The listing builds one solid part. Answer for the finished solid, in the listing's coordinates (mm). Face numbers are marked on the shaded views. A direction names the side the tool comes from. Give positions to 0.01 mm unless a question says otherwise; leave off trailing zeros. Loops run counter-clockwise (first coordinate to the right, second up) from the corner with the lowest first, then second, coordinate; pieces in that order, holes last. Notation, with made-up numbers: M 79.25,87 L 131.25,87 A16 cw 131.25,100 Z; hole C 78,57.25 d3. An arc over 180 degrees is marked long. One line per item, written item: value. Start each with the question number.
Q1. The mould has two halves that part along X. Classify the marked faces 4, 5 and 6: +X half, -X half, draft (parallel to the pull), parting line (faces both ways), or undercut.
Q2. Consider L1, parallel to X at y = 36.25, z = -0.65; L2, parallel to Y at x = 0.25, z = 1.6; L3, parallel to X at y = 29.5, z = -0.15. Determine where each line is inside the solid, lowest interval first.
Q3. For the marked faces 1, 2 and 3, determine the directions among +Z, -Z, +X, -X, +Y, -Y from which every point of the face is accessible in a straight line to the end or side of a thin tool.
Q4. A cutting plane is placed at B-B, the plane y = 28.75. Determine the outline of the cut face in (x, z), and give its area (3 significant figures).
Q5. A cutting plane is placed at A-A, the plane z = 0. Determine the outline of the cut face in (x, y) (3 decimals), and give its area (3 significant figures).
Q6. Flat-ended cylindrical pins translate along their axes: pin 1 (0.9 mm diameter, centred on y = 28, z = 0, fed in from +X); pin 2 (0.9 mm diameter, centred on y = 36.5, z = -1, fed in from -X); pin 3 (3 mm diameter, centred on y = 28.5, z = 0.5, fed in from -X). Find the tip coordinate at first contact, or state that the pin passes through.
Q7. A cutting plane is placed at C-C, the plane y = 32.75. Determine the outline of the cut face in (x, z).
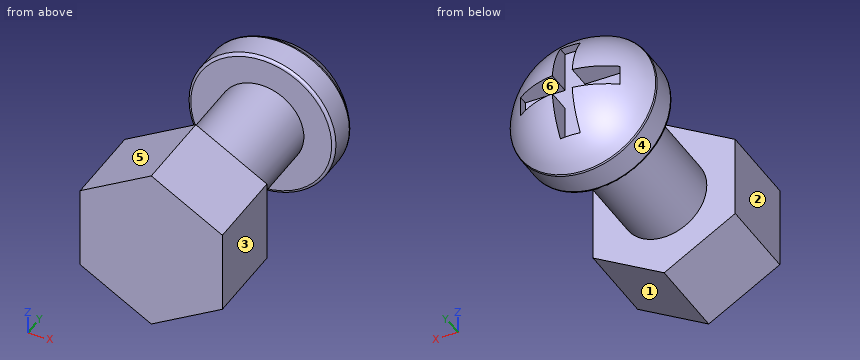
from build123d import *

# Parameters (mm, degrees)
SKETCH1_R           = 1.5
BOSS_EXTRUDE1_DEPTH = 30
SKETCH1_4_R         = 1.5
BOSS_EXTRUDE2_DEPTH = 6
SKETCH4_W           = 0.7
SKETCH4_H           = 1.4
SKETCH4_W_2         = 1.4
SKETCH4_H_2         = 0.7
CUT_EXTRUDE1_DEPTH  = 4
FILLET1_R           = 0.1
SKETCH5_R           = 1.5
BOSS_EXTRUDE3_DEPTH = 3
SKETCH6_R           = 4.535168768
CUT_EXTRUDE2_DEPTH  = 33


with BuildPart() as part:
    # Sketch1 → Boss-Extrude1 (new body)
    # profile 1 of 2: a face of its own
    with BuildSketch(Plane(origin=(0, 0, 0), x_dir=(1, 0, 0), z_dir=(0, 1, 0))):
        Polygon((0, -2.886751346), (2.5, -1.443375673), (2.5, 1.443375673), (0, 2.886751346), (-2.5, 1.443375673), (-2.5, -1.443375673), align=None)
        Circle(SKETCH1_R, mode=Mode.SUBTRACT)
    # profile 2 of 2: a face of its own
    with BuildSketch(Plane(origin=(0, 0, 0), x_dir=(1, 0, 0), z_dir=(0, 1, 0))):
        Circle(SKETCH1_R)
    extrude(amount=BOSS_EXTRUDE1_DEPTH)

    # Sketch1_4 → Boss-Extrude2 (add)
    with BuildSketch(Plane(origin=(0, 0, 0), x_dir=(1, 0, 0), z_dir=(0, 1, 0))):
        with Locations(Location((0, 0, 0), (0, 0, 270))):
            Circle(SKETCH1_4_R)
    extrude(amount=-BOSS_EXTRUDE2_DEPTH)

    # Sketch3 one side → Revolve1 (revolve)
    with BuildSketch(Plane.XY, mode=Mode.PRIVATE) as revolve1_sk:
        with BuildLine():
            Line((0, 36.9), (0, 30.9))
            Line((0, 30.9), (0, 30))
            Line((0, 30), (1.5, 30))
            Line((1.5, 30), (1.5, 34.4))
            Line((1.5, 34.4), (2.577677109, 34.4))
            Line((2.577677109, 34.4), (2.577677109, 35.4))
            ThreePointArc((2.577677109, 35.4), (2.572999105, 35.433876498), (2.559315235, 35.465217406))
            ThreePointArc((2.559315235, 35.465217406), (1.467028933, 36.516835132), (0, 36.9))
        make_face()
    revolve(revolve1_sk.sketch.rotate(Axis((0, 30, 0), (0, -1, 0)), 180), axis=Axis((0, 30, 0), (0, -1, 0)))

    # Sketch4 → Cut-Extrude1 (cut)
    with BuildSketch(Plane(origin=(0, 40, 0), x_dir=(1, 0, 0), z_dir=(0, 1, 0))):
        with Locations((0, -1.05)):
            Rectangle(SKETCH4_W, SKETCH4_H)
        with Locations((1.05, 0)):
            Rectangle(SKETCH4_W_2, SKETCH4_H_2)
        with Locations((0, 1.05)):
            Rectangle(SKETCH4_W, SKETCH4_H)
        with Locations((-1.05, 0)):
            Rectangle(SKETCH4_W_2, SKETCH4_H_2)
        Rectangle(SKETCH4_W, SKETCH4_H_2)
    extrude(amount=-CUT_EXTRUDE1_DEPTH, mode=Mode.SUBTRACT)

    # Fillet1
    fillet1_edges = [part.edges().sort_by_distance(p)[0] for p in [
        (2.577677109, 34.4, 0),
    ]]
    fillet(fillet1_edges, radius=FILLET1_R)


with BuildPart() as body_2:
    # Sketch5 → Boss-Extrude3 (new body)
    with BuildSketch(Plane.XZ.offset(6)):
        Polygon((2.5, 1.443375673), (0, 2.886751346), (-2.5, 1.443375673), (-2.5, -1.443375673), (0, -2.886751346), (2.5, -1.443375673), align=None)
        with Locations(Location((0, 0, 0), (0, 0, 90))):
            Circle(SKETCH5_R, mode=Mode.SUBTRACT)
    extrude(amount=-BOSS_EXTRUDE3_DEPTH)


with BuildPart() as cut_extrude2_tool:
    # Sketch6 → Cut-Extrude2 (new body)
    with BuildSketch(Plane.XZ.offset(6)):
        Circle(SKETCH6_R)
    extrude(amount=-CUT_EXTRUDE2_DEPTH)


with BuildPart() as part_1:
    add(part.part)

    # Cut-Extrude2: cut by cut_extrude2_tool
    add(cut_extrude2_tool.part, mode=Mode.SUBTRACT)


with BuildPart() as body_2_1:
    add(body_2.part)

    # Cut-Extrude2: cut by cut_extrude2_tool
    add(cut_extrude2_tool.part, mode=Mode.SUBTRACT)


solid = part_1.part
Answer block:
1. face 4: parting line
1. face 5: -X half
1. face 6: undercut
2. L1: -1.75 to -0.35, 0.35 to 1.75
2. L2: 27 to 30, 34.4 to 36
2. L3: -2.5 to 2.5
3. face 1: -Z, +X, -Y
3. face 2: +Z, -Z, -X, -Y
3. face 3: +Z, -Z, +X, -Y
4. outline: M -2.5,-1.44 L 0,-2.89 L 2.5,-1.44 L 2.5,1.44 L 0,2.89 L -2.5,1.44 Z
4. area: 21.7 mm^2
5. outline: M -2.578,34.5 A0.1 ccw -2.478,34.4 L -1.5,34.4 L -1.5,30 L -2.5,30 L -2.5,27 L 2.5,27 L 2.5,30 L 1.5,30 L 1.5,34.4 L 2.478,34.4 A0.1 ccw 2.578,34.5 L 2.578,35.4 A0.125 ccw 2.559,35.465 A3 ccw 1.75,36.337 L 1.75,36 L -1.75,36 L -1.75,36.337 A3 ccw -2.559,35.465 A0.125 ccw -2.578,35.4 Z
5. area: 36.4 mm^2
6. pin 1: x = 2.5
6. pin 2: x = -1.88
6. pin 3: x = -2.5
7. outline: C 0,0 d3
